Job drawing, mm, ordinate dimensions from the low corner. One solid piece. A direction names the side the tool comes from. Round coordinates to 2 decimals unless told otherwise and drop trailing zeros. Write each loop counter-clockwise with the first axis right and the second up, starting at its lowest first coordinate (ties: lowest second). Pieces come first, ordered by that corner, then holes.
1) Flat gauge pins, fed straight in: pin 1 (8 mm diameter, centred on x = 15.5, z = 8.5, fed in from +Y); pin 2 (3 mm diameter, centred on x = 34.5, y = 31, fed in from +Z); pin 3 (8 mm diameter, centred on x = 7.5, z = 25.5, fed in from -Y). Where does each tip first touch, or does it go through?
2) Saw through at D-D on x = 34. Write the cut outline in (y, z), and give its area (3 significant figures).
3) Saw through at B-B on y = 8. Write the cut outline in (x, z).
4) Saw through at A-A on z = 19.5. Write the cut outline in (x, y), and give its area (3 significant figures).
5) Saw through at C-C on x = 25. Write the cut outline in (y, z).
6) Drill centre lines: L1, parallel to X at y = 8, z = 40.4; L2, parallel to X at y = 20.6, z = 19.5; L3, parallel to X at y = 21, z = 19. Where is each one in solid material? Low to high.
7) Which spindle directions (+Z, -Z, +X, -X, +Y, -Y) get a long thin tool onto all of the face, cutting with end or side? Do the marked faces 1, 2 and 3. Say none if no direction does.
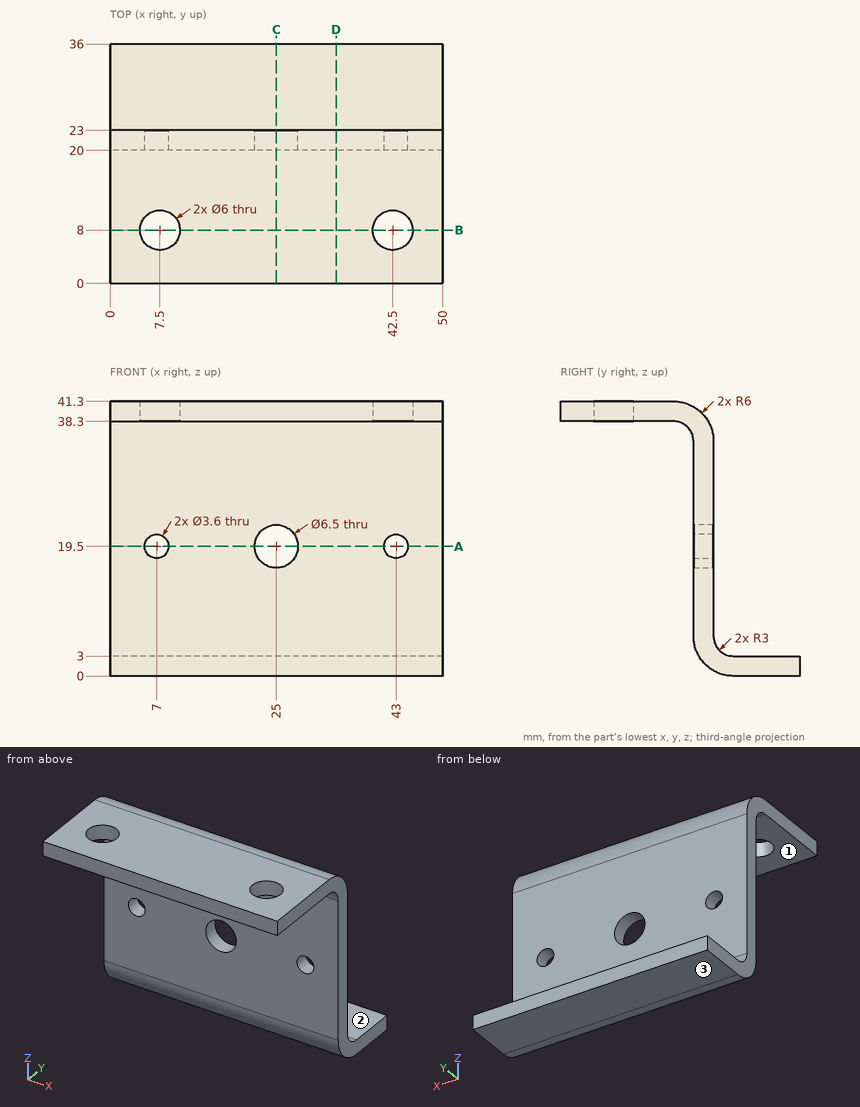
Completed:
1. pin 1: stops at y = 23.4
1. pin 2: stops at z = 3
1. pin 3: stops at y = 20
2. outline: (0, 38.3) - (17, 38.3) arc R3 cw to (20, 35.3) - (20, 6) arc R6 ccw to (26, 0) - (36, 0) - (36, 3) - (26, 3) arc R3 cw to (23, 6) - (23, 35.3) arc R6 ccw to (17, 41.3) - (0, 41.3) - close
2. area: 211 mm2
3. outline: (0, 38.3) - (4.5, 38.3) - (4.5, 41.3) - (0, 41.3) - close; (10.5, 38.3) - (39.5, 38.3) - (39.5, 41.3) - (10.5, 41.3) - close; (45.5, 38.3) - (50, 38.3) - (50, 41.3) - (45.5, 41.3) - close
4. outline: (0, 20) - (5.2, 20) - (5.2, 23) - (0, 23) - close; (8.8, 20) - (21.75, 20) - (21.75, 23) - (8.8, 23) - close; (28.25, 20) - (41.2, 20) - (41.2, 23) - (28.25, 23) - close; (44.8, 20) - (50, 20) - (50, 23) - (44.8, 23) - close
4. area: 109 mm2
5. outline: (0, 38.3) - (17, 38.3) arc R3 cw to (20, 35.3) - (20, 22.75) - (23, 22.75) - (23, 35.3) arc R6 ccw to (17, 41.3) - (0, 41.3) - close; (20, 6) arc R6 ccw to (26, 0) - (36, 0) - (36, 3) - (26, 3) arc R3 cw to (23, 6) - (23, 16.25) - (20, 16.25) - close
6. L1: x = 0 to 4.5, 10.5 to 39.5, 45.5 to 50
6. L2: x = 0 to 5.2, 8.8 to 21.75, 28.25 to 41.2, 44.8 to 50
6. L3: x = 0 to 5.27, 8.73 to 21.79, 28.21 to 41.27, 44.73 to 50
7. face 1: -Z, +X, -X, -Y
7. face 2: +Z, +X, -X, +Y
7. face 3: -Z, +X, -X, +Y, -Y
